CAD build for the part. Positions are in the model's coordinates, mm. A direction names the side the tool comes from. Coordinates: 2 decimals unless noted, no trailing zeros. Order: outer loops, then holes, each group sorted by start corner. A loop starts at its lowest first (then second) coordinate and runs counter-clockwise, first axis right, second up. Notation, with made-up numbers: (-39.75, 36.5) - (-18.75, 36.5) arc R16 cw to (-18.75, 49.5) - close; hole circle Ø3 at (64.5, 30.5). An arc over 180 degrees is marked (long way). Write each question's results on one line, items separated by ' | '. Start each with the question number.
Q1. Band-saw the part on C-C, the plane z = -4. Write the cut outline in (x, y), then the cut area to 3 significant figures.
Q2. Wall check: probe 1 along X at (y, z) = (-1.05, -5); probe 2 along Z at (x, y) = (-7.5, 0.7); probe 3 along Z at (x, y) = (11, 0.95). Give the ranges that are in metal, low to high.
Q3. Band-saw the part on B-B, the plane y = -0.7. Write the cut outline in (x, z), then the cut area to 3 significant figures.
Q4. Band-saw the part on A-A, the plane x = 8.5. Write the cut outline in (y, z).
Q5. Which spindle directions (+Z, -Z, +X, -X, +Y, -Y) get a long thin tool onto all of the face, cutting with end or side? Do faces 5 (the flat face through (0, 0, 20.7)), 6 (the flat face through (-19.7, 0, 6)). Say none if no direction does.
Q6. Pull direction Z, two halves, no side cores. Call faces 1 (the flat face through (0, 0, -18.7)), 2 (the cylindrical face through (16.72, 0.02, -16.56)), 3 (the flat face through (0, 0, 21.7)), 4 (the flat face through (18.7, 0, 6)): released by +Z, released by -Z, zero draft, split by the parting line, or undercut.
```python
from build123d import *

# Parameters (mm, degrees)
BOSS_EXTRUDE1_DEPTH = 1.5
FILLET1_R           = 1


with BuildPart() as part:
    # Sketch1 → Boss-Extrude1 (new, symmetric)
    with BuildSketch(Plane(origin=(0, 0, 0), x_dir=(1, 0, 0), z_dir=(0, 1, 0))):
        with BuildLine():
            Line((-19.7, 9.25), (-19.7, -21.7))
            Line((-19.7, -21.7), (19.7, -21.7))
            Line((19.7, -21.7), (19.7, 9.25))
            ThreePointArc((19.7, 9.25), (16.639265863, 16.639265863), (9.25, 19.7))
            Line((9.25, 19.7), (-9.25, 19.7))
            ThreePointArc((-9.25, 19.7), (-16.639265863, 16.639265863), (-19.7, 9.25))
        make_face()
        with BuildLine():
            Line((-18.7, -20.7), (18.7, -20.7))
            Line((18.7, -20.7), (18.7, 9.25))
            ThreePointArc((18.7, 9.25), (15.932159082, 15.932159082), (9.25, 18.7))
            Line((9.25, 18.7), (-9.25, 18.7))
            ThreePointArc((-9.25, 18.7), (-15.932159082, 15.932159082), (-18.7, 9.25))
            Line((-18.7, 9.25), (-18.7, -20.7))
        make_face(mode=Mode.SUBTRACT)
    extrude(amount=BOSS_EXTRUDE1_DEPTH, both=True)

    # Fillet1
    fillet1_edges = [part.edges().sort_by_distance(p)[0] for p in [
        (19.7, 0, 21.7),
        (-19.7, 0, 21.7),
    ]]
    fillet(fillet1_edges, radius=FILLET1_R)


solid = part.part
```
Results below:
1) outline: (-19.7, -1.5) - (-18.7, -1.5) - (-18.7, 1.5) - (-19.7, 1.5) - close; (18.7, -1.5) - (19.7, -1.5) - (19.7, 1.5) - (18.7, 1.5) - close | area: 6.00 mm²
2) probe 1: x = -19.7 to -18.7, 18.7 to 19.7 | probe 2: z = -19.7 to -18.7, 20.7 to 21.7 | probe 3: z = -19.55 to -18.54, 20.7 to 21.7
3) outline: (-19.7, -9.25) arc R10.45 ccw to (-9.25, -19.7) - (9.25, -19.7) arc R10.45 ccw to (19.7, -9.25) - (19.7, 20.7) arc R1 ccw to (18.7, 21.7) - (-18.7, 21.7) arc R1 ccw to (-19.7, 20.7) - close; hole (-18.7, -9.25) arc R9.45 ccw to (-9.25, -18.7) - (9.25, -18.7) arc R9.45 ccw to (18.7, -9.25) - (18.7, 20.7) - (-18.7, 20.7) - close | area: 149 mm²
4) outline: (-1.5, -19.7) - (1.5, -19.7) - (1.5, -18.7) - (-1.5, -18.7) - close; (-1.5, 20.7) - (1.5, 20.7) - (1.5, 21.7) - (-1.5, 21.7) - close
5) face 5: +Y, -Y | face 6: +Z, -Z, -X, +Y, -Y
6) face 1: undercut | face 2: released by -Z | face 3: released by +Z | face 4: undercut
